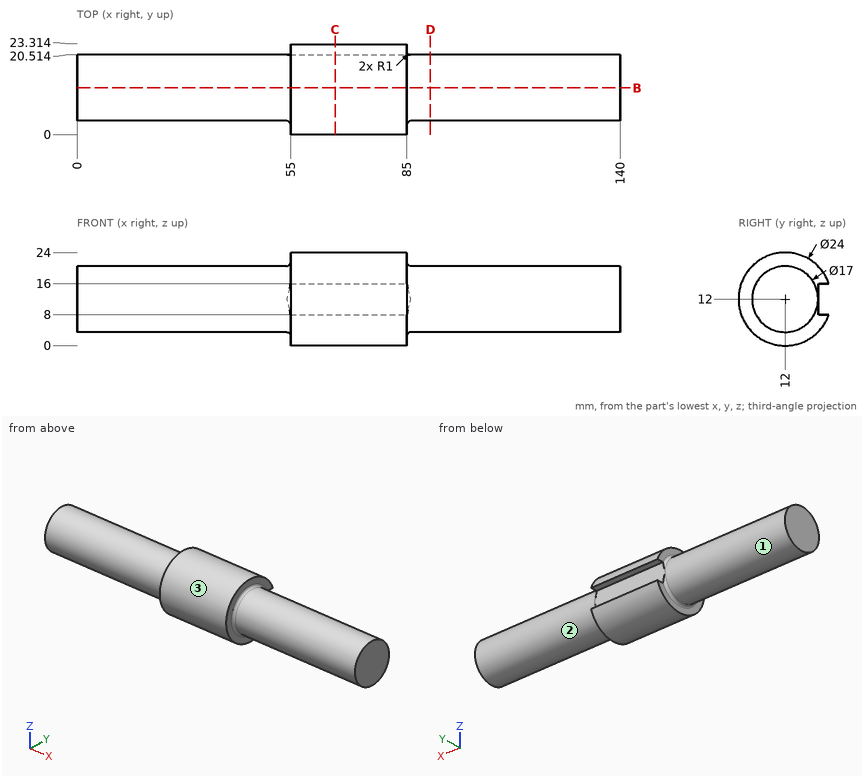
Part print with two shaded views. Sizes in mm from the minimum x, y, z corner. A direction names the side the tool comes from. Coordinates: 2 decimals unless noted, no trailing zeros. Order: outer loops, then holes, each group sorted by start corner. A loop starts at its lowest first (then second) coordinate and runs counter-clockwise, first axis right, second up.
(1) Saw through at B-B, the plane y = 12. Write the cut outline in (x, z), and give its area (3 significant figures).
Solution:
outline: (0, 3.5) - (54, 3.5) arc R1 cw to (55, 2.5) - (55, 0) - (85, 0) - (85, 2.5) arc R1 cw to (86, 3.5) - (140, 3.5) - (140, 20.5) - (86, 20.5) arc R1 cw to (85, 21.5) - (85, 24) - (55, 24) - (55, 21.5) arc R1 cw to (54, 20.5) - (0, 20.5) - close
area: 2,590 mm2
(2) Pin check, flat tips, straight feed: pin 1 Ø0.8 at (x, y) = (66, 22) entering from -Z; pin 2 Ø3 at (x, z) = (24.5, 17) entering from +Y; pin 3 Ø10 at (x, z) = (114.5, 13.5) entering from -Y. Stop position of each tip, or through.
Solution:
pin 1: stops at z = 4.8
pin 2: stops at y = 19.75
pin 3: stops at y = 3.5
(3) Drill centre lines: L1, parallel to X at y = 2, z = 8.75; L2, parallel to Z at x = 70, y = 12.75; L3, parallel to Y at x = 8, z = 14.5 (1 decimal). Where is each one in solid material? Low to high.
Solution:
L1: x = 55 to 85
L2: z = 0.02 to 23.98
L3: y = 3.9 to 20.1
(4) Saw through at D-D, the plane x = 91. Write the cut outline in (y, z), and give its area (3 significant figures).
Solution:
outline: circle Ø17 at (12, 12)
area: 227 mm2
(5) Saw through at C-C, the plane x = 66.5. Write the cut outline in (y, z), and give its area (3 significant figures).
Solution:
outline: (20.51, 8) - (20.51, 16) - (23.31, 16) arc R12 ccw (long way) to (23.31, 8) - close
area: 426 mm2
(6) Which spindle directions (+Z, -Z, +X, -X, +Y, -Y) get a long thin tool onto all of the face, cutting with end or side? Do the marked faces 1, 2 and 3. Say none if no direction does.
Solution:
face 1: -X
face 2: +X
face 3: +X, -X
